Build history of the part. All positions in model axes, mm. Face numbers are marked on the shaded views. A direction names the side the tool comes from. Give positions to 0.01 mm unless a question says otherwise; leave off trailing zeros. Order: outer loops, then holes, each group sorted by start corner. A loop starts at its lowest first (then second) coordinate and runs counter-clockwise, first axis right, second up. Notation, with made-up numbers: (45, 63.25) - (93, 63.25) arc R17 ccw to (93, 81.25) - close; hole circle Ø9 at (23, 11). An arc over 180 degrees is marked (long way). Answer in a Markdown table with one row per item.
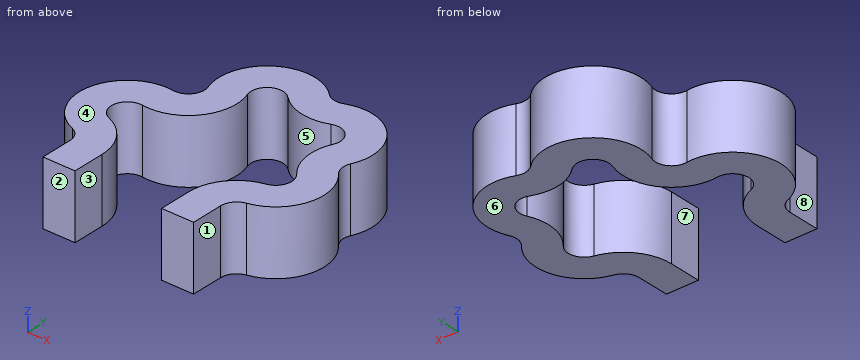
Autodesk Inventor part; units mm, degrees
ref_plane "YZ Plane" through (0, 0, 0) normal (1, 0, 0) x (0, 1, 0)
ref_plane "XY Plane" through (0, 0, 0) normal (0, 0, 1) x (1, 0, 0)
sketch "Sketch1" plane through (0, 0, 0) normal (0, 0, 1) x (1, 0, 0)
  line L0 (0.85, 11.55) -> (0.85, -11.55) construction
  arc A0 (0.85, 11.55) -> (-0.85, 11.55) centre (0, 11.55) ccw construction
  line L1 (-0.85, -11.55) -> (-0.85, 11.55) construction
  arc A1 (-0.85, -11.55) -> (0.85, -11.55) centre (0, -11.55) ccw construction
  line L2 (-2.85, 11.55) -> (-2.85, -6.75) construction
  arc A2 (-2.85, 11.55) -> (-4.55, 11.55) centre (-3.7, 11.55) ccw construction
  line L3 (-4.55, -6.75) -> (-4.55, 11.55) construction
  arc A3 (-4.55, -6.75) -> (-2.85, -6.75) centre (-3.7, -6.75) ccw construction
  line L4 (0, 12.4) -> (0, 13.4)
  line L5 (-3.7, 12.4) -> (-3.7, 13.4)
  arc A4 (0.7872, 14.3771) -> (0, 13.4) centre (1, 13.4) ccw
  arc A5 (0.7872, 14.3771) -> (1.3256, 16.0142) centre (0.5744, 15.3542) ccw
  arc A6 (1.1707, 17.0972) -> (1.3256, 16.0142) centre (2.0769, 16.6743) ccw
  arc A7 (1.1707, 17.0972) -> (-0.1098, 18.4474) centre (0.2645, 17.5201) ccw
  arc A8 (-1.1733, 18.65) -> (-0.1098, 18.4474) centre (-0.4842, 19.3746) ccw
  arc A9 (-3.7, 13.4) -> (-4.3417, 14.3336) centre (-4.7, 13.4) ccw
  arc A10 (-3.8648, 16.2602) -> (-4.3417, 14.3336) centre (-3.9835, 15.2672) ccw
  arc A11 (-3.8648, 16.2602) -> (-2.8042, 17.5892) centre (-3.746, 17.2531) ccw
  arc A12 (-1.1733, 18.65) -> (-2.8042, 17.5892) centre (-1.8624, 17.9253) ccw
  point P0 (0, 0)
  dimension "d0" = 1
  dimension "d1" = 1
  dimension "d2" = 1
  dimension "d3" = 1
  dimension "d4" = 1
  dimension "d5" = 1
  dimension "d6" = 1
  dimension "d7" = 1
  dimension "d8" = 1
  dimension "d9" = 1
  dimension "d10" = 1
ref_plane "Work Plane1" through (-3.7, 12.4, 0) normal (0, 1, 0) x (-1, 0, 0)
sketch "Sketch2" plane through (-3.7, 12.4, 0) normal (0, 1, 0) x (-1, 0, 0)
  line L0 (-0.5, 0) -> (0.5, 0)
  line L1 (0.5, 0) -> (0.5, -2)
  line L2 (0.5, -2) -> (-0.5, -2)
  line L3 (-0.5, -2) -> (-0.5, 0)
  point P0 (-3.7, 0)
  point P1 (0, 0)
  dimension "d11" = 1
  dimension "d12" = 2
sweep "Sweep1" add profiles "Sketch2" path "Sketch1"
properties part number "string2"
1. Drop flat-ended pins along their axis: P1, Ø0.8, axis at y = 13, z = -1.5, coming from the +X side; P2, Ø4, axis at x = -3, y = 17, coming from the +Z side; P3, Ø0.5, axis at y = 13, z = -1.5, coming from the -X side. Give the stop position or say it passes through.
Check result:
| item | result |
|---|---|
| P1 | stops at x = 0.5 |
| P2 | stops at z = 0 |
| P3 | stops at x = -4.2 |
2. Probe line 1 (X direction, y = 15, z = -1); line 2 (X direction, y = 13.5, z = -1.35); line 3 (Y direction, x = -5, z = -0.1). List the from-to ranges inside material, lowest first.
Check result:
| item | result |
|---|---|
| line 1 | x = -5.46 to -4.41, 0.93 to 2.03 |
| line 2 | x = -4.21 to -3.2, -0.5 to 0.51 |
| line 3 | y = 14.16 to 16.37 |
3. Cut at C-C on y = 14. Write the cut outline in (x, z).
Check result:
| item | result |
|---|---|
| outline | (-4.79, -2) - (-3.33, -2) - (-3.33, 0) - (-4.79, 0) - close; (-0.37, -2) - (1.22, -2) - (1.22, 0) - (-0.37, 0) - close |
4. Cut at A-A on y = 13.25. Write the cut outline in (x, z), and give its area (3 significant figures).
Check result:
| item | result |
|---|---|
| outline | (-4.2, -2) - (-3.2, -2) - (-3.2, 0) - (-4.2, 0) - close; (-0.5, -2) - (0.5, -2) - (0.5, 0) - (-0.5, 0) - close |
| area | 4.00 mm² |
5. Cut at B-B on z = -0.3. Write the cut outline in (x, y), and give its area (3 significant figures).
Check result:
| item | result |
|---|---|
| outline | (-4.52, 13.87) arc R0.5 cw to (-4.2, 13.4) - (-4.2, 12.4) - (-3.2, 12.4) - (-3.2, 13.4) arc R1.5 ccw to (-4.16, 14.8) arc R0.5 cw to (-3.92, 15.76) arc R1.5 ccw to (-2.33, 17.76) arc R0.5 cw to (-1.52, 18.29) arc R1.5 ccw to (0.08, 17.98) arc R0.5 cw to (0.72, 17.31) arc R1.5 ccw to (0.95, 15.68) arc R0.5 cw to (0.68, 14.87) arc R1.5 ccw to (-0.5, 13.4) - (-0.5, 12.4) - (0.5, 12.4) - (0.5, 13.4) arc R0.5 cw to (0.89, 13.89) arc R1.5 ccw to (1.7, 16.34) arc R0.5 cw to (1.62, 16.89) arc R1.5 ccw to (-0.3, 18.91) arc R0.5 cw to (-0.83, 19.01) arc R1.5 ccw to (-3.28, 17.42) arc R0.5 cw to (-3.81, 16.76) arc R1.5 ccw to start |
| area | 18.9 mm² |
6. Which spindle directions (+Z, -Z, +X, -X, +Y, -Y) get a long thin tool onto all of the face, cutting with end or side? Do the marked faces 1, 2, 3, 4 and 5. Say none if no direction does.
Check result:
| item | result |
|---|---|
| face 1 | +Z, -Z, +X, -Y |
| face 2 | +Z, -Z, +X, -X, -Y |
| face 3 | +Z, -Z, -Y |
| face 4 | +Z, +X, -X, +Y, -Y |
| face 5 | +Z, -Z |
7. Two-plate mould, pull along X, no slides. Class the marked faces 6, 7 and 8: +X half, -X half, draft (parallel to the pull), parting line (faces both ways), or undercut.
Check result:
| item | result |
|---|---|
| face 6 | draft |
| face 7 | undercut |
| face 8 | -X half |
